Check sheet for the modelled part. Datum: model origin and axes. Units: mm. Round coordinates to 2 decimals unless told otherwise and drop trailing zeros. Loops run counter-clockwise (first coordinate to the right, second up) from the corner with the lowest first, then second, coordinate; pieces in that order, holes last. Notation, with made-up numbers: (36, -7.75) - (85, -7.75) arc R22 ccw to (85, 15.25) - close; hole circle Ø10 at (-40, -25.75). An arc over 180 degrees is marked (long way). Put each result on its own line as item: value. Start each with the question number.
Item 1: Gauge pin test, flat ends, axial feed: pin 1 Ø1.8 at (x, z) = (-38.5, 24) entering from +Y; pin 2 Ø10 at (y, z) = (9, 8) entering from -X; pin 3 Ø12 at (x, y) = (-33.5, 6) entering from -Z. Record the tip position at first contact, or that the pin passes through.
Item 2: Section check A-A, the plane y = 8.75. Record the cut outline in (x, z).
Item 3: Section check C-C, the plane x = -39. Record the cut outline in (y, z).
Item 4: Section check B-B, the plane z = 20.5. Record the cut outline in (x, y).
Item 5: Material ranges on line 1 along X through (y, z) = (-2.75, -21); line 2 along Y through (x, z) = (-34, -7), recorded low to high.
Item 6: Section check D-D, the plane z = -24.5. Record the cut outline in (x, y).
from build123d import *

# Parameters (mm, degrees)
BOX_W         = 91.62
BOX_H         = 2.5
BOX_DEPTH     = 60.3
SKETCH_R      = 2
PAD_DEPTH     = 3
SKETCH001_W   = 22.1
SKETCH001_H   = 60.3
SKETCH001_W_2 = 14
SKETCH001_H_2 = 16.304
PAD001_DEPTH  = 2.5
SKETCH002_R   = 1.1
PAD002_DEPTH  = 2.5


with BuildPart() as part:
    # Box → Box (new body)
    with BuildSketch(Plane(origin=(-45.5, -6.5, -29), x_dir=(1, 0, 0), z_dir=(0, 0, 1))):
        with Locations((45.81, 1.25)):
            Rectangle(BOX_W, BOX_H)
    extrude(amount=BOX_DEPTH)

    # Sketch → Pad (new body)
    with BuildSketch(Plane(origin=(-45.5, -4, -29), x_dir=(-1, 0, 0), z_dir=(0, 1, 0))):
        with Locations((-6.5, 4.5)):
            Circle(SKETCH_R)
        with Locations((-64.5, 4.5)):
            Circle(SKETCH_R)
        with Locations((-64.5, 53.5)):
            Circle(SKETCH_R)
        with Locations((-6.5, 53.5)):
            Circle(SKETCH_R)
    extrude(amount=PAD_DEPTH)

    # Sketch001 → Pad001 (new body)
    with BuildSketch(Plane(origin=(46.12, -6.5, -29), x_dir=(0, 1, 0), z_dir=(1, 0, 0))):
        with Locations((11.05, 30.15)):
            Rectangle(SKETCH001_W, SKETCH001_H)
        with Locations((13.5, 46.348)):
            Rectangle(SKETCH001_W_2, SKETCH001_H_2, mode=Mode.SUBTRACT)
    extrude(amount=PAD001_DEPTH)

    # Sketch002 → Pad002 (new body)
    with BuildSketch(Plane(origin=(-45.5, -1, -29), x_dir=(-1, 0, 0), z_dir=(0, 1, 0))):
        with Locations((-64.5, 4.5)):
            Circle(SKETCH002_R)
        with Locations((-64.5, 53.5)):
            Circle(SKETCH002_R)
        with Locations((-6.5, 53.5)):
            Circle(SKETCH002_R)
        with Locations((-6.5, 4.5)):
            Circle(SKETCH002_R)
    extrude(amount=PAD002_DEPTH)


solid = part.part
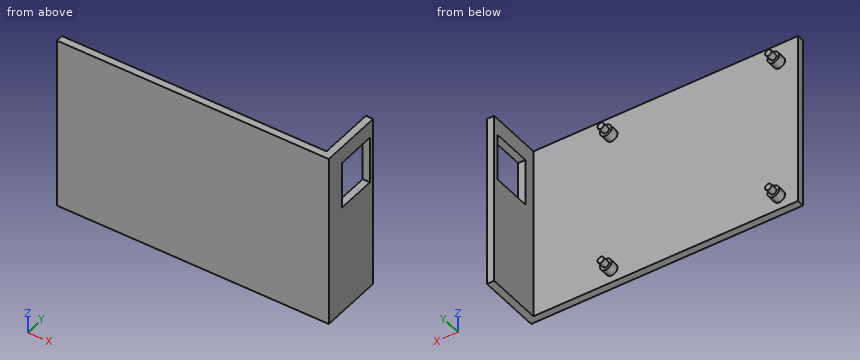
Check result:
1. pin 1: y = 1.5
1. pin 2: x = 46.12
1. pin 3: through
2. outline: (46.12, -29) - (48.62, -29) - (48.62, 9.2) - (46.12, 9.2) - close; (46.12, 25.5) - (48.62, 25.5) - (48.62, 31.3) - (46.12, 31.3) - close
3. outline: (-6.5, -29) - (-4, -29) - (-4, -26.5) - (-1, -26.5) - (-1, -25.6) - (1.5, -25.6) - (1.5, -23.4) - (-1, -23.4) - (-1, -22.5) - (-4, -22.5) - (-4, 22.5) - (-1, 22.5) - (-1, 23.4) - (1.5, 23.4) - (1.5, 25.6) - (-1, 25.6) - (-1, 26.5) - (-4, 26.5) - (-4, 31.3) - (-6.5, 31.3) - close
4. outline: (-45.5, -6.5) - (48.62, -6.5) - (48.62, 0) - (46.12, 0) - (46.12, -4) - (-45.5, -4) - close; (46.12, 14) - (48.62, 14) - (48.62, 15.6) - (46.12, 15.6) - close
5. line 1: 46.12 to 48.62
5. line 2: -6.5 to -4
6. outline: (-45.5, -6.5) - (48.62, -6.5) - (48.62, 15.6) - (46.12, 15.6) - (46.12, -4) - (21, -4) - (21, -1) - (20.1, -1) - (20.1, 1.5) - (17.9, 1.5) - (17.9, -1) - (17, -1) - (17, -4) - (-37, -4) - (-37, -1) - (-37.9, -1) - (-37.9, 1.5) - (-40.1, 1.5) - (-40.1, -1) - (-41, -1) - (-41, -4) - (-45.5, -4) - close
